```python
from build123d import *

# Parameters (mm, degrees)
DODANIE_WYCI_GNI_CIE1_DEPTH = 350
SZKIC2_W                    = 140.103855023
SZKIC2_H                    = 128.958798703
WYTNIJ_WYCI_GNI_CIE1_DEPTH  = 297.057426862
SZKIC3_W                    = 180.28107172
SZKIC3_H                    = 138.969006622
WYTNIJ_WYCI_GNI_CIE2_DEPTH  = 327.955654485


with BuildPart() as part:
    # Szkic1 → Dodanie-wyciągnięcie1 (new body)
    with BuildSketch(Plane.XY):
        with BuildLine():
            ThreePointArc((0, 57), (0.878679656, 59.121320344), (3, 60))
            Line((3, 60), (57, 60))
            ThreePointArc((57, 60), (59.121320344, 59.121320344), (60, 57))
            Line((60, 57), (60, 3))
            ThreePointArc((60, 3), (59.121320344, 0.878679656), (57, 0))
            Line((57, 0), (3, 0))
            ThreePointArc((3, 0), (0.878679656, 0.878679656), (0, 3))
            Line((0, 3), (0, 57))
        make_face()
        with BuildLine():
            Line((3, 6), (3, 54))
            ThreePointArc((3, 54), (3.878679656, 56.121320344), (6, 57))
            Line((6, 57), (54, 57))
            ThreePointArc((54, 57), (56.121320344, 56.121320344), (57, 54))
            Line((57, 54), (57, 6))
            ThreePointArc((57, 6), (56.121320344, 3.878679656), (54, 3))
            Line((54, 3), (6, 3))
            ThreePointArc((6, 3), (3.878679656, 3.878679656), (3, 6))
        make_face(mode=Mode.SUBTRACT)
    extrude(amount=DODANIE_WYCI_GNI_CIE1_DEPTH)

    # Szkic2 → Wytnij-wyciągnięcie1 (cut, through all)
    with BuildSketch(Plane(origin=(0, -145, 145), x_dir=(1, 0, 0), z_dir=(0, -0.7071067811865488, 0.7071067811865464))):
        with Locations((39.65073467, 253.465731554)):
            Rectangle(SZKIC2_W, SZKIC2_H)
    extrude(amount=WYTNIJ_WYCI_GNI_CIE1_DEPTH, mode=Mode.SUBTRACT)

    # Szkic3 → Wytnij-wyciągnięcie2 (cut, through all)
    with BuildSketch(Plane(origin=(0, 30, 30), x_dir=(1, 0, 0), z_dir=(0, -0.7071067811865488, -0.7071067811865464))):
        with Locations((27.094402169, -5.623479723)):
            Rectangle(SZKIC3_W, SZKIC3_H)
    extrude(amount=WYTNIJ_WYCI_GNI_CIE2_DEPTH, mode=Mode.SUBTRACT)


solid = part.part
```
Source: CAD feature listing. Evaluate the final solid. Frame: model axes, mm. A direction names the side the tool comes from. Round coordinates to 2 decimals unless told otherwise and drop trailing zeros. Write each loop counter-clockwise with the first axis right and the second up, starting at its lowest first coordinate (ties: lowest second). Pieces come first, ordered by that corner, then holes. Notation, with made-up numbers: M 45,-14.75 L 66,-14.75 A15 cw 66,8.25 Z; hole C -8,77.5 d6. An arc over 180 degrees is marked long. Answer as a JSON object with one key per item and string values. Group by question number.
(1) Ray query, line 1 (X direction, y = 33, z = 179); line 2 (Y direction, x = 21.5, z = 58.5). Return the intervals inside material, ascending. Write a range as [from, to].
(2) Section query A-A on y = 29.5. Output: boundary loops of the cut face in (x, z).
(3) Section query C-C on z = 44. Output: boundary loops of the cut face in (x, y), then the cut area to 3 significant figures.
(4) Mould query, pull axis X, two halves, no side actions, for faces 1 (the flat face through (30, 3, 173)), 2 (the flat face through (0, 30, 173)), 3 (the flat face through (1, 32, 322)). Classes: +X half, -X half, draft (parallel to the pull), parting line (faces both ways), or undercut.
(5) Section query B-B on x = 14.5. Output: boundary loops of the cut face in (y, z).
(6) Section query D-D on z = 218. Output: boundary loops of the cut face in (x, y).
(7) Reachability of faces 4 (the flat face through (57, 30, 173)), 5 (the flat face through (30, 0, 173)) from +Z, -Z, +X, -X, +Y, -Y: full face, straight path, thin tool, end or side. Return the list, or none.
Computed values:
{
 "1": {"line 1": "[0, 3], [57, 60]", "line 2": "[1.5, 3], [57, 60]"},
 "2": {"outline": "M 0,30.5 L 3,30.5 L 3,319.5 L 0,319.5 Z; M 57,30.5 L 60,30.5 L 60,319.5 L 57,319.5 Z"},
 "3": {"outline": "M 0,16 L 3,16 L 3,54 A3 cw 6,57 L 54,57 A3 cw 57,54 L 57,16 L 60,16 L 60,57 A3 ccw 57,60 L 3,60 A3 ccw 0,57 Z", "area": "426 mm^2"},
 "4": {"face 1": "undercut", "face 2": "-X half", "face 3": "draft"},
 "5": {"outline": "M 0,60 L 3,57 L 3,293 L 0,290 Z; M 57,3 L 60,0 L 60,350 L 57,347 Z"},
 "6": {"outline": "M 0,3 A3 ccw 3,0 L 57,0 A3 ccw 60,3 L 60,57 A3 ccw 57,60 L 3,60 A3 ccw 0,57 Z; hole M 3,6 A3 ccw 6,3 L 54,3 A3 ccw 57,6 L 57,54 A3 ccw 54,57 L 6,57 A3 ccw 3,54 Z"},
 "7": {"face 4": "+Z, -Z", "face 5": "+Z, -Z, +X, -X, -Y"}
}
